Source: CAD feature listing. Evaluate the final solid. Frame: model axes, mm. Face numbers are marked on the shaded views. Give positions to 0.01 mm unless a question says otherwise; leave off trailing zeros. Write each loop counter-clockwise with the first axis right and the second up, starting at its lowest first coordinate (ties: lowest second). Pieces come first, ordered by that corner, then holes. Notation, with made-up numbers: M 24,-15 L 59,-15 A25 ccw 59,10 Z; hole C 8,86 d5. An arc over 180 degrees is marked long. Use CSV: the item, a comma, the result in double quotes. Start each with the question number.
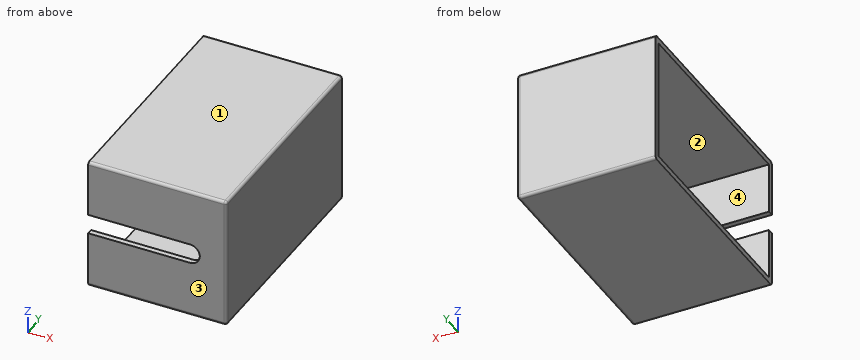
Autodesk Fusion 360 part; units mm, degrees
sketch "Sketch1" plane through (0, 0, 0) normal (1, 0, 0) x (0, 1, 0) in component "Box"
  line L0 (0, 0) -> (80, 0)
  line L1 (80, 0) -> (80, 47)
  line L2 (80, 47) -> (0, 47)
  line L3 (0, 47) -> (0, 0)
  dimension "d1" = 80
  dimension "d2" = 47
extrude "Extrude1" add sketch "Sketch1" along normal blind 49 in component "Box"
sketch "Sketch2" plane through (0, 0, 0) normal (-1, 0, 0) x (0, -1, 0) in component "Box"
  line L0 (0, 0) -> (0, 47)
  line L1 (0, 47) -> (-80, 47)
  line L2 (-80, 47) -> (-80, 0)
  line L3 (-80, 0) -> (0, 0)
  line L4 (-78, 2) -> (-2, 2)
  line L5 (-2, 2) -> (-2, 45)
  line L6 (-2, 45) -> (-78, 45)
  line L7 (-78, 45) -> (-78, 2)
  dimension "d5" = -2
extrude "Extrude2" cut sketch "Sketch2" against normal blind 47 contours L4 L5 L6 L7 in component "Box"
sketch "Sketch3" plane through (0, 0, 0) normal (0, 1, 0) x (1, 0, 0) in component "Box"
  circle A0 centre (36, -23.5) radius 3.5
  line L0 (0, -47) -> (0, 0)
  line L1 (0, 0) -> (49, 0)
  line L2 (36, -20) -> (0, -20)
  line L3 (36, -27) -> (0, -27)
  dimension "d8" = 7
  dimension "d12" = 36
  dimension "d13" = 23.5
extrude "Extrude3" cut sketch "Sketch3" along normal up to surface (2 mm away) in component "Box"
fillet "Fillet1" radius 1 8 edges at (24.5, 0, 47) (24.5, 80, 47) (24.5, 80, 0) (24.5, 0, 0) (49, 40, 47) (49, 40, 0) (49, 0, 23.5) (49, 80, 23.5) in component "Box"
component "Box" placed x (1, 0, 0) y (0, 1, 0) z (0, 0, 1) at (0, 0, 0)
Item 1: Pull-direction query (Z, two-part tool) for the marked faces 1, 2, 3 and 4; classes: released by +Z, released by -Z, zero draft, split by the parting line, or undercut.
Item 2: Section D-D (x = 38). Return the cut outline in (y, z).
Item 3: Section C-C (x = 28.5). Return the cut outline in (y, z).
Item 4: Section A-A (z = 33.5). Return the cut outline in (x, y), plus the area to 3 significant figures.
Item 5: Contact query for a flat-ended pin moving along its axis: pin 1 Ø10 at (y, z) = (63.5, 36) entering from -X. Output: stop coordinate, or through.
Item 6: Material intervals for probe 1 along Z at (x, y) = (22.5, 27); probe 2 along Y at (x, z) = (41.5, 21); probe 3 along X at (y, z) = (46, 7), sorted ascending.
Item 7: Section B-B (y = 54.5). Return the cut outline in (x, z), plus the area to 3 significant figures.
Output values:
1,face 1,"released by +Z"
1,face 2,"undercut"
1,face 3,"zero draft"
1,face 4,"undercut"
2,outline,"M 0,1 A1 ccw 1,0 L 79,0 A1 ccw 80,1 L 80,46 A1 ccw 79,47 L 1,47 A1 ccw 0,46 L 0,26.37 L 2,26.37 L 2,45 L 78,45 L 78,2 L 2,2 L 2,20.63 L 0,20.63 Z"
3,outline,"M 0,1 A1 ccw 1,0 L 79,0 A1 ccw 80,1 L 80,46 A1 ccw 79,47 L 1,47 A1 ccw 0,46 L 0,27 L 2,27 L 2,45 L 78,45 L 78,2 L 2,2 L 2,20 L 0,20 Z"
4,outline,"M 0,0 L 48,0 A1 ccw 49,1 L 49,79 A1 ccw 48,80 L 0,80 L 0,78 L 47,78 L 47,2 L 0,2 Z"
4,area,"348 mm2"
5,pin 1,"stops at x = 47"
6,probe 1,"z = 0 to 2, 45 to 47"
6,probe 2,"y = 0 to 2, 78 to 80"
6,probe 3,"x = 47 to 49"
7,outline,"M 0,0 L 48,0 A1 ccw 49,1 L 49,46 A1 ccw 48,47 L 0,47 L 0,45 L 47,45 L 47,2 L 0,2 Z"
7,area,"282 mm2"
